Could you check a few things on this model? Use its own coordinates, in mm. Face numbers are marked on the shaded views. A direction names the side the tool comes from. Give positions to 0.01 mm unless a question says otherwise; leave off trailing zeros. Order: outer loops, then holes, each group sorted by start corner. A loop starts at its lowest first (then second) coordinate and runs counter-clockwise, first axis right, second up.
(1) Will these pins go through, and if not, where does the flat tip stop? pin 1 (1.5 mm diameter, centred on x = -24.5, y = 22.5, fed in from +Z); pin 2 (5 mm diameter, centred on x = 0, z = 0, fed in from -Y) (3 decimals); pin 3 (5 mm diameter, centred on y = 26.5, z = -28.5, fed in from +X); pin 4 (1 mm diameter, centred on x = 6.5, y = 16.5, fed in from +Z).
(2) Imagine slicing it at B-B, the plane x = 0. Write out the boundary of the cut face in (y, z) (3 decimals).
(3) Imagine slicing it at A-A, the plane z = 0. Write out the boundary of the cut face in (x, y) (3 decimals).
(4) Imagine slicing it at D-D, the plane y = 6. Write out the boundary of the cut face in (x, z) (3 decimals), then the cut area to 3 significant figures.
(5) Imagine slicing it at C-C, the plane y = 20.75. Write out the boundary of the cut face in (x, z) (3 decimals), then the cut area to 3 significant figures.
(6) On a 3-axis mill with a long thin cutter (end or side, diameter ignored), from which of +Z, -Z, +X, -X, +Y, -Y can I reach the whole of each face in a straight line? I mean the marked faces 1 and 2. Say none if no direction works.
(7) If I drill on probe 1 along X at (y, z) = (27.8, 0) (3 decimals); probe 2 along Y at (x, z) = (-1, -22), over which ranges is the centre line in solid material (lowest first)?
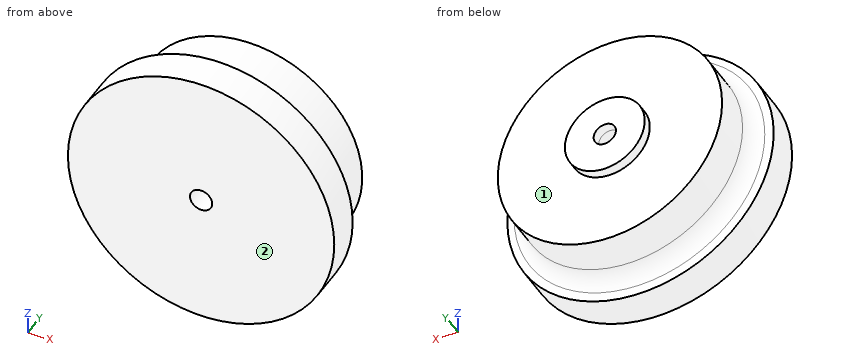
from build123d import *

# Parameters (mm, degrees)
F_1_4_0_25_DIAMETER_HOLE1_D = 6.35
SKETCH3_R                   = 11.3792
SKETCH3_R_2                 = 3.175
BOSS_EXTRUDE1_DEPTH         = 2.794


with BuildPart() as part:
    # Sketch1 → Revolve1 (revolve)
    with BuildSketch(Plane.XY, mode=Mode.PRIVATE) as revolve1_sk:
        with BuildLine():
            Line((0, 0), (37.973, 0))
            Line((37.973, 0), (37.973, 10.0076))
            Line((37.973, 10.0076), (35.750149251, 10.603211063))
            ThreePointArc((35.750149251, 10.603211063), (33.034715031, 12.417606201), (31.98495, 15.510114261))
            Line((31.98495, 15.510114261), (31.98495, 26.67))
            Line((31.98495, 26.67), (0, 26.67))
            Line((0, 26.67), (0, 0))
        make_face()
    revolve(revolve1_sk.sketch.rotate(Axis((0, 26.67, 0), (0, -1, 0)), 180), axis=Axis((0, 26.67, 0), (0, -1, 0)))

    # 1/4 (0.25) Diameter Hole1 (through all)
    with Locations(Plane(origin=(0, 26.67, 0), x_dir=(1, 0, 0), z_dir=(0, 1, 0))):
        with Locations((0, 0)):
            Hole(F_1_4_0_25_DIAMETER_HOLE1_D / 2)

    # Sketch3 → Boss-Extrude1 (add)
    with BuildSketch(Plane(origin=(0, 26.67, 0), x_dir=(1, 0, 0), z_dir=(0, 1, 0))):
        Circle(SKETCH3_R)
        with Locations(Location((0, 0, 0), (0, 0, 270))):
            Circle(SKETCH3_R_2, mode=Mode.SUBTRACT)
    extrude(amount=BOSS_EXTRUDE1_DEPTH)


solid = part.part
Answer block:
1. pin 1: stops at z = 21.42
1. pin 2: passes through
1. pin 3: stops at x = 18.63
1. pin 4: stops at z = 31.42
2. outline: (0, -37.973) - (10.008, -37.973) - (10.603, -35.75) arc R5.08 cw to (15.51, -31.985) - (26.67, -31.985) - (26.67, -11.379) - (29.464, -11.379) - (29.464, -3.175) - (0, -3.175) - close; (0, 3.175) - (29.464, 3.175) - (29.464, 11.379) - (26.67, 11.379) - (26.67, 31.985) - (15.51, 31.985) arc R5.08 cw to (10.603, 35.75) - (10.008, 37.973) - (0, 37.973) - close
3. outline: (-37.973, 0) - (-3.175, 0) - (-3.175, 29.464) - (-11.379, 29.464) - (-11.379, 26.67) - (-31.985, 26.67) - (-31.985, 15.51) arc R5.08 cw to (-35.75, 10.603) - (-37.973, 10.008) - close; (3.175, 0) - (37.973, 0) - (37.973, 10.008) - (35.75, 10.603) arc R5.08 cw to (31.985, 15.51) - (31.985, 26.67) - (11.379, 26.67) - (11.379, 29.464) - (3.175, 29.464) - close
4. outline: circle Ø75.946 at (0, 0); hole circle Ø6.35 at (0, 0)
4. area: 4,500 mm2
5. outline: circle Ø63.97 at (0, 0); hole circle Ø6.35 at (0, 0)
5. area: 3,180 mm2
6. face 1: +Y
6. face 2: +Z, -Z, +X, -X, -Y
7. probe 1: x = -11.379 to -3.175, 3.175 to 11.379
7. probe 2: y = 0 to 26.67
